Geometry: final body of the model. Coordinates: model frame, mm. A direction names the side the tool comes from. Coordinates: 2 decimals unless noted, no trailing zeros. Write each loop counter-clockwise with the first axis right and the second up, starting at its lowest first coordinate (ties: lowest second). Pieces come first, ordered by that corner, then holes. Notation, with made-up numbers: (3, 83) - (23, 83) arc R13 ccw to (23, 90) - close; hole circle Ø4 at (29.5, 74). An arc over 180 degrees is marked (long way). Answer as a JSON object with one key per item and string values. Group by question number.
Item 1: Line query: line 1 along Z through (x, y) = (3.5, -0.6); line 2 along X through (y, z) = (1.2, -28.55); line 3 along X through (y, z) = (-0.45, 28.55). Output: solid intervals per line, ascending. Write a range as from..to.
Item 2: First-contact query: pin 1 Ø5.5 at (x, z) = (3.45, 28.55) entering from +Y (3 decimals). Flat tip, straight axial feed; report the tip coordinate or a pass-through.
Item 3: Section C-C on x = 10.75. Return loops of the section in (y, z) (3 decimals).
Item 4: Section A-A on z = 28.55. Return loops of the section in (x, y) (3 decimals).
Item 5: Section D-D on z = -27.5. Return loops of the section in (x, y) (3 decimals).
Item 6: Section B-B on y = -0.55. Return loops of the section in (x, z).
Item 7: Mould query, pull axis X, two halves, no side actions, for faces 1 (the flat face through (2, 0.425, 30)), 2 (the flat face through (2, 0.425, -27)), 3 (the flat face through (15, 1, 0)), 4 (the flat face through (7, 1.625, 0)). Classes: pulls with the +X half, pulls with the -X half, needs draft (parallel to the pull), parting line crosses it, or undercut.
Item 8: Set-up query: faces 5 (the cylindrical face through (2.39, -0.59, -29.94)), 6 (the flat face through (7, -1, 25)), 7 (the cylindrical face through (4.4, 1, -25.6)). Return all of +Z, -Z, +X, -X, +Y, -Y with unobstructed straight access to the full face (end or side cutting, diameter ignored); none if empty.
```python
from build123d import *

# Parameters (mm, degrees)
EXTRUDE_1_DEPTH     = 15
SKETCH_2_R          = 1.75
CUT_EXTRUDE_1_DEPTH = 37.394539426
SKETCH_2_3_R        = 3.1
SKETCH_2_3_R_2      = 1.75
CUT_EXTRUDE_2_DEPTH = 1.2


with BuildPart() as part:
    # Sketch 1 → Extrude 1 (new body)
    with BuildSketch(Plane(origin=(0, 0, 0), x_dir=(0, 0, -1), z_dir=(1, 0, 0))):
        Polygon((33, 1.625), (-33, 1.625), (-33, -1.625), (-25, -1.625), (-25, 0.375), (1, 0.375), (1, -1.625), (33, -1.625), align=None)
    extrude(amount=EXTRUDE_1_DEPTH)

    # Sketch 2 → Cut-Extrude 1 (cut, through all)
    with BuildSketch(Plane(origin=(0, 1.625, 0), x_dir=(1, 0, 0), z_dir=(0, 1, 0))):
        with Locations(Location((3.451122219, -28.55, 0), (0, 0, 270))):
            Circle(SKETCH_2_R)
        with Locations(Location((3.451122219, 28.55, 0), (0, 0, 270))):
            Circle(SKETCH_2_R)
    extrude(amount=-CUT_EXTRUDE_1_DEPTH, mode=Mode.SUBTRACT)

    # Sketch 2_3 → Cut-Extrude 2 (cut)
    # profile 1 of 2: a face of its own
    with BuildSketch(Plane(origin=(0, 1.625, 0), x_dir=(1, 0, 0), z_dir=(0, 1, 0))):
        with Locations(Location((3.451122219, 28.55, 0), (0, 0, 270))):
            Circle(SKETCH_2_3_R)
        with Locations(Location((3.451122219, 28.55, 0), (0, 0, 270))):
            Circle(SKETCH_2_3_R_2, mode=Mode.SUBTRACT)
    # profile 2 of 2: a face of its own
    with BuildSketch(Plane(origin=(0, 1.625, 0), x_dir=(1, 0, 0), z_dir=(0, 1, 0))):
        with Locations(Location((3.451122219, -28.55, 0), (0, 0, 270))):
            Circle(SKETCH_2_3_R)
        with Locations(Location((3.451122219, -28.55, 0), (0, 0, 270))):
            Circle(SKETCH_2_3_R_2, mode=Mode.SUBTRACT)
    extrude(amount=-CUT_EXTRUDE_2_DEPTH, mode=Mode.SUBTRACT)


solid = part.part
```
Checks:
{
 "1": {"line 1": "-33..-30.3, -26.8..-1, 25..26.8, 30.3..33", "line 2": "0..0.35, 6.55..15", "line 3": "0..1.7, 5.2..15"},
 "2": {"pin 1": "y = 0.425"},
 "3": {"outline": "(-1.625, -33) - (1.625, -33) - (1.625, 33) - (-1.625, 33) - (-1.625, 25) - (0.375, 25) - (0.375, -1) - (-1.625, -1) - close"},
 "4": {"outline": "(0, -1.625) - (1.701, -1.625) - (1.701, 0.425) - (0.351, 0.425) - (0.351, 1.625) - (0, 1.625) - close; (5.201, -1.625) - (15, -1.625) - (15, 1.625) - (6.551, 1.625) - (6.551, 0.425) - (5.201, 0.425) - close"},
 "5": {"outline": "(0, -1.625) - (2.051, -1.625) - (2.051, 0.425) - (0.534, 0.425) - (0.534, 1.625) - (0, 1.625) - close; (4.851, -1.625) - (15, -1.625) - (15, 1.625) - (6.368, 1.625) - (6.368, 0.425) - (4.851, 0.425) - close"},
 "6": {"outline": "(0, -33) - (15, -33) - (15, -1) - (0, -1) - close; (0, 25) - (15, 25) - (15, 33) - (0, 33) - close; hole circle Ø3.5 at (3.45, -28.55); hole circle Ø3.5 at (3.45, 28.55)"},
 "7": {"face 1": "undercut", "face 2": "undercut", "face 3": "pulls with the +X half", "face 4": "needs draft"},
 "8": {"face 5": "+Y, -Y", "face 6": "+X, -X, -Y", "face 7": "+Y"}
}
